from build123d import *

# Parameters (mm, degrees)
ESQUISSE1_W             = 60
ESQUISSE1_H             = 40
BOSS_EXTRU_1_DEPTH      = 9
ESQUISSE2_W             = 25
ESQUISSE2_H             = 40
ESQUISSE2_W_2           = 6
ENL_V_MAT_EXTRU_1_DEPTH = 7
ESQUISSE3_R             = 2
ENL_V_MAT_EXTRU_2_DEPTH = 54.907327888
ESQUISSE4_W             = 3
ESQUISSE4_H             = 32
ENL_V_MAT_EXTRU_3_DEPTH = 73.449982747
CONG_1_R                = 3


with BuildPart() as part:
    # Esquisse1 → Boss.-Extru.1 (new body)
    with BuildSketch(Plane.XY):
        with Locations((30, 20)):
            Rectangle(ESQUISSE1_W, ESQUISSE1_H)
    extrude(amount=BOSS_EXTRU_1_DEPTH)

    # Esquisse2 → Enlèv. mat.-Extru.1 (cut)
    with BuildSketch(Plane(origin=(0, 0, 0), x_dir=(-1, 0, 0), z_dir=(0, 0, -1))):
        with Locations((-12.5, 20)):
            Rectangle(ESQUISSE2_W, ESQUISSE2_H)
        with Locations((-47.5, 20)):
            Rectangle(ESQUISSE2_W, ESQUISSE2_H)
        with Locations((-30, 20)):
            Rectangle(ESQUISSE2_W_2, ESQUISSE2_H)
    extrude(amount=-ENL_V_MAT_EXTRU_1_DEPTH, mode=Mode.SUBTRACT)

    # Esquisse3 → Enlèv. mat.-Extru.2 (cut, through all)
    with BuildSketch(Plane(origin=(35, 0, 0), x_dir=(0, 0, -1), z_dir=(1, 0, 0))):
        with Locations((-3.5, 5)):
            Circle(ESQUISSE3_R)
        with Locations((-3.5, 35)):
            Circle(ESQUISSE3_R)
    extrude(amount=-ENL_V_MAT_EXTRU_2_DEPTH, mode=Mode.SUBTRACT)

    # Esquisse4 → Enlèv. mat.-Extru.3 (cut, through all)
    with BuildSketch(Plane(origin=(0, 0, 7), x_dir=(-1, 0, 0), z_dir=(0, 0, -1))):
        with Locations((-47.5, 20)):
            Rectangle(ESQUISSE4_W, ESQUISSE4_H)
        with Locations((-54.5, 20)):
            Rectangle(ESQUISSE4_W, ESQUISSE4_H)
        with Locations((-40.5, 20)):
            Rectangle(ESQUISSE4_W, ESQUISSE4_H)
        with Locations((-12.5, 20)):
            Rectangle(ESQUISSE4_W, ESQUISSE4_H)
        with Locations((-5.5, 20)):
            Rectangle(ESQUISSE4_W, ESQUISSE4_H)
        with Locations((-19.5, 20)):
            Rectangle(ESQUISSE4_W, ESQUISSE4_H)
    extrude(amount=-ENL_V_MAT_EXTRU_3_DEPTH, mode=Mode.SUBTRACT)

    # Congé1
    cong_1_edges = [part.edges().sort_by_distance(p)[0] for p in [
        (0, 40, 8),
        (60, 40, 8),
        (60, 0, 8),
        (0, 0, 8),
    ]]
    fillet(cong_1_edges, radius=CONG_1_R)


solid = part.part
The model under review builds one solid part; all positions refer to its coordinate system, in mm. A direction names the side the tool comes from. Round coordinates to 2 decimals unless told otherwise and drop trailing zeros. Loops run counter-clockwise (first coordinate to the right, second up) from the corner with the lowest first, then second, coordinate; pieces in that order, holes last. Notation, with made-up numbers: (2.5, 45.5) -> (12.5, 45.5) arc R22 cw to (12.5, 84.5) -> close; hole circle Ø7 at (-9.75, 14). An arc over 180 degrees is marked (long way). One line per question, with ' | ' between items. Start each with the question number.
Item 1: Add section A-A, the plane z = 3.5. Write out the cut boundary in (x, y), then the cut area to 3 significant figures.
Item 2: Add section D-D, the plane x = 10. Write out the cut boundary in (y, z), then the cut area to 3 significant figures.
Item 3: Add section C-C, the plane y = 35. Count the separate pieces of the cut face and the enclosed holes in it, then the cut area to 3 significant figures.
Item 4: Draft analysis for pull direction Z (two halves, no side actions). For faces 1 (the face through (34.014, 33.048, 3.934)), 2 (the face through (30, 20, 7)), 3 (the face through (34.014, 6.352, 4.974)), 4 (the face through (55, 4, 8)), state which applies: +Z half, -Z half, draft (parallel to the pull), parting line (faces both ways), or undercut.
Item 5: Machinability: for faces 5 (the face through (0.86, 39.1, 8.01)), 6 (the face through (27, 20, 3)), 7 (the face through (53, 20, 8)), which of the approach directions +Z, -Z, +X, -X, +Y, -Y give a long, thin tool a straight path to every point of the face, cutting with its end or side? Answer none if there is none.
Item 6: Wall thickness on line 1 along Y through (x, z) = (25.6, 3.5); line 2 along X through (y, z) = (24, 6.5); line 3 along Y through (x, z) = (34.5, 1.75): over which ranges is each line inside the solid? List them lowest first. Write a range as [from, to].
Item 7: Add section B-B, the plane x = 20. Write out the cut boundary in (y, z), then the cut area to 3 significant figures.
Item 8: For pin 1 (2 mm diameter, centred on y = 25.5, z = 5, fed in from +X); pin 2 (5 mm diameter, centred on x = 31, y = 24, fed in from -Z); pin 3 (5 mm diameter, centred on x = 48, y = 18.5, fed in from -Z); pin 4 (3 mm diameter, centred on y = 7.5, z = 1, fed in from -X), all flat-tipped, find the tip position at first contact; note any pin that passes through.
Return value:
1) outline: (25, 0) -> (27, 0) -> (27, 3) -> (25, 3) -> close; (25, 7) -> (27, 7) -> (27, 33) -> (25, 33) -> close; (25, 37) -> (27, 37) -> (27, 40) -> (25, 40) -> close; (33, 0) -> (35, 0) -> (35, 3) -> (33, 3) -> close; (33, 7) -> (35, 7) -> (35, 33) -> (33, 33) -> close; (33, 37) -> (35, 37) -> (35, 40) -> (33, 40) -> close | area: 128 mm2
2) outline: (0, 7) -> (40, 7) -> (40, 9) -> (0, 9) -> close | area: 80.0 mm2
3) separate pieces: 9 | enclosed holes: 0 | area: 96.0 mm2
4) face 1: undercut | face 2: -Z half | face 3: undercut | face 4: draft
5) face 5: +Z, -Z, -X, +Y | face 6: -Z, +Y, -Y | face 7: +Z, -Z
6) line 1: y = [0, 3], [7, 33], [37, 40] | line 2: x = [25, 27], [33, 35] | line 3: y = [0, 4.03], [5.97, 34.03], [35.97, 40]
7) outline: (0, 7) -> (4, 7) -> (4, 9) -> (0, 9) -> close; (36, 7) -> (40, 7) -> (40, 9) -> (36, 9) -> close | area: 16.0 mm2
8) pin 1: stops at x = 35 | pin 2: stops at z = 0 | pin 3: stops at z = 7 | pin 4: stops at x = 25
